The listing builds one solid part. Answer for the finished solid, in the listing's coordinates (mm). Coordinates: 2 decimals unless noted, no trailing zeros. Order: outer loops, then holes, each group sorted by start corner. A loop starts at its lowest first (then second) coordinate and runs counter-clockwise, first axis right, second up. Notation, with made-up numbers: (-5.5, 56) -> (30.5, 56) arc R18 cw to (30.5, 60) -> close; hole circle Ø10 at (88, 51). An arc over 180 degrees is marked (long way). Answer in a Markdown table with one row per item. Add a question column.
Autodesk Inventor part; units mm, degrees
ref_plane "YZ Plane" through (0, 0, 0) normal (1, 0, 0) x (0, 1, 0)
ref_plane "XZ Plane" through (0, 0, 0) normal (0, 1, 0) x (-1, 0, 0)
ref_plane "XY Plane" through (0, 0, 0) normal (0, 0, 1) x (1, 0, 0)
sketch "Sketch1" plane through (0, 0, 0) normal (1, 0, 0) x (0, 1, 0)
  line L0 (1.5875, 12.7) -> (-1.5875, 12.7)
  line L1 (-1.5875, 12.7) -> (-1.5875, -12.7)
  line L2 (-1.5875, -12.7) -> (1.5875, -12.7)
  line L3 (1.5875, -12.7) -> (1.5875, 12.7)
  line L4 (1.5875, 12.7) -> (-1.5875, -12.7) construction
  line L5 (-1.5875, 12.7) -> (1.5875, -12.7) construction
  point P0 (0, 0)
  dimension "d0" = 3.175
  dimension "d1" = 25.4
extrude "Extrusion1" add sketch "Sketch1" along normal mid plane 60
sketch "Sketch2" plane through (-30, 1.5875, 12.7) normal (0, 1, 0) x (1, 0, 0)
  line L0 (0, 0) -> (0, 25.4)
  line L1 (0, 12.7) -> (34.5, 12.7)
  line L2 (34.5, 12.7) -> (254.5, 12.7)
  circle A0 centre (34.5, 12.7) radius 2.5
  circle A1 centre (254.5, 12.7) radius 2.5
  point P0 (30, 12.7)
  dimension "d4" = 34.5
  dimension "d5" = 220
  dimension "d6" = 5
  dimension "d7" = 5
extrude "Extrusion2" cut sketch "Sketch2" against normal blind 250 contours A0 L2 L1 | L1 L2 A0
properties part number "PLETINA PARA CARA INCLINADA"
Q1. A cutting plane is placed at A-A (x = 4.5). Determine the outline of the cut face in (y, z).
Q2. A cutting plane is placed at B-B (z = 0). Determine the outline of the cut face in (x, y), then the cut area to 3 significant figures.
Q3. Determine the mould class of faces 1 (the face through (0, 0, 12.7)), 2 (the face through (6.885, 0.022, -0.751)), 3 (the face through (0, -1.588, 0)), 4 (the face through (0, 0, -12.7)) for opening direction Z: +Z half, -Z half, draft (parallel to the pull), parting line (faces both ways), or undercut.
Q4. Straight lines are drawn through the part: line 1 (Z direction, x = 4.5, y = -0.65); line 2 (X direction, y = 1.45, z = 0); line 3 (Z direction, x = 5, y = 0.1). For each, find the intervals that lie inside material, in ascending order.
Returned:
| question | item | result |
|---|---|---|
| 1 | outline | (-1.59, -12.7) -> (1.59, -12.7) -> (1.59, -2.5) -> (-1.59, -2.5) -> close; (-1.59, 2.5) -> (1.59, 2.5) -> (1.59, 12.7) -> (-1.59, 12.7) -> close |
| 2 | outline | (-30, -1.59) -> (2, -1.59) -> (2, 1.59) -> (-30, 1.59) -> close; (7, -1.59) -> (30, -1.59) -> (30, 1.59) -> (7, 1.59) -> close |
| 2 | area | 175 mm² |
| 3 | face 1 | +Z half |
| 3 | face 2 | undercut |
| 3 | face 3 | draft |
| 3 | face 4 | -Z half |
| 4 | line 1 | z = -12.7 to -2.5, 2.5 to 12.7 |
| 4 | line 2 | x = -30 to 2, 7 to 30 |
| 4 | line 3 | z = -12.7 to -2.45, 2.45 to 12.7 |
